from build123d import *

# Parameters (mm, degrees)
ESBO_O1_R                  = 10
ESBO_O1_R_2                = 9
RESSALTO_EXTRUS_O1_DEPTH   = 5.5
CORTE_EXTRUS_O1_REACH      = 25.66
ESBO_O2_R                  = 2.25
ESBO_O3_R                  = 2.25
CORTE_EXTRUS_O2_DEPTH      = 11.0000001
CORTE_EXTRUS_O2_DEPTH_BACK = 11.0000001


with BuildPart() as part:
    # Esboço1 → Ressalto-extrusão1 (new body, symmetric)
    with BuildSketch(Plane(origin=(0, 0, 0), x_dir=(1, 0, 0), z_dir=(0, 1, 0))):
        Circle(ESBO_O1_R)
        Circle(ESBO_O1_R_2, mode=Mode.SUBTRACT)
    extrude(amount=RESSALTO_EXTRUS_O1_DEPTH, both=True)

    # Esboço2 → Corte-extrusão1 (cut, up to next)
    with BuildSketch(Plane(origin=(-8.660254038, 0, -5), x_dir=(-0.5, 0, 0.866025404), z_dir=(-0.866025404, 0, -0.5)), mode=Mode.PRIVATE) as corte_extrus_o1_sk1:
        Circle(ESBO_O2_R)
    corte_extrus_o1_tool1 = extrude(corte_extrus_o1_sk1.sketch, amount=-CORTE_EXTRUS_O1_REACH, mode=Mode.PRIVATE) & part.part
    add(corte_extrus_o1_tool1.solids().sort_by_distance((-8.660254, 0, -5))[0], mode=Mode.SUBTRACT)

    # Esboço3 → Corte-extrusão2 (cut, two sides)
    with BuildSketch(Plane(origin=(0, 0, 0), x_dir=(0, 0, -1), z_dir=(1, 0, 0))) as corte_extrus_o2_sk:
        Circle(ESBO_O3_R)
    extrude(amount=CORTE_EXTRUS_O2_DEPTH, mode=Mode.SUBTRACT)
    extrude(corte_extrus_o2_sk.sketch, amount=-CORTE_EXTRUS_O2_DEPTH_BACK, mode=Mode.SUBTRACT)


solid = part.part
The model under review builds one solid part; all positions refer to its coordinate system, in mm. Coordinates: 2 decimals unless noted, no trailing zeros. Loops run counter-clockwise (first coordinate to the right, second up) from the corner with the lowest first, then second, coordinate; pieces in that order, holes last. Notation, with made-up numbers: M -18,64 L -11,64 A11 cw -11,69 Z; hole C 23.5,-32.5 d1. An arc over 180 degrees is marked long. Put each result on its own line as item: value. Start each with the question number.
Q1. Add section C-C (y = 0). Write out the cut boundary in (x, z).
Q2. The part is to be moulded in two halves that separate along Y. For faces 1 (the cylindrical face through (-9.348, 0.676, -2.146)), 2 (the flat face through (-9, -5.5, -2)), 3 (the flat face through (-9, 5.5, -2)), say which applies: +Y half, -Y half, draft (parallel to the pull), parting line (faces both ways), or undercut.
Q3. Add section D-D (z = 6.25). Write out the cut boundary in (x, y).
Q4. Add section B-B (z = 0). Write out the cut boundary in (x, y).
Q5. Clearance check with flat-ended pins moving along their axes: pin 1 (2 mm diameter, centred on y = 4, z = 5.5, fed in from +X); pin 2 (5 mm diameter, centred on y = 2.5, z = -3.5, fed in from +X); pin 3 (1 mm diameter, centred on y = 1.5, z = 2, fed in from -X); pin 4 (4 mm diameter, centred on y = 0, z = 0, fed in from -X). State where each tip first meets the part, or that it passes through.
Q6. Add section A-A (x = 0). Write out the cut boundary in (y, z), and give its area (3 significant figures).
Q7. Wall thickness on line 1 (Y direction, x = 9.45, z = 0); line 2 (Z direction, x = 2.75, y = -2.25); line 3 (Z direction, x = 4, y = 5.25): over which ranges is each line inside the solid? List them lowest first.
Answers:
1. outline: M -9.74,-2.25 A10 ccw -9.56,-2.92 L -8.67,-2.41 A9 cw -8.71,-2.25 Z; M -9.74,2.25 L -8.71,2.25 A9 cw 8.71,2.25 L 9.74,2.25 A10 ccw Z; M -7.31,-6.82 A10 ccw 9.74,-2.25 L 8.71,-2.25 A9 cw -6.42,-6.31 Z
2. face 1: undercut
2. face 2: -Y half
2. face 3: +Y half
3. outline: M -7.81,-5.5 L -6.48,-5.5 L -6.48,5.5 L -7.81,5.5 Z; M 6.48,-5.5 L 7.81,-5.5 L 7.81,5.5 L 6.48,5.5 Z
4. outline: M -10,-5.5 L -9,-5.5 L -9,-2.25 L -10,-2.25 Z; M -10,2.25 L -9,2.25 L -9,5.5 L -10,5.5 Z; M 9,-5.5 L 10,-5.5 L 10,-2.25 L 9,-2.25 Z; M 9,2.25 L 10,2.25 L 10,5.5 L 9,5.5 Z
5. pin 1: stops at x = 8.93
5. pin 2: stops at x = 9.95
5. pin 3: stops at x = -9.88
5. pin 4: passes through
6. outline: M -5.5,-10 L 5.5,-10 L 5.5,-9 L -5.5,-9 Z; M -5.5,9 L 5.5,9 L 5.5,10 L -5.5,10 Z
6. area: 22.0 mm^2
7. line 1: y = -5.5 to -2.25, 2.25 to 5.5
7. line 2: z = -9.61 to -8.57, 8.57 to 9.61
7. line 3: z = -9.17 to -8.06, 8.06 to 9.17
